The listing builds one solid part. Answer for the finished solid, in the listing's coordinates (mm). A direction names the side the tool comes from. Round coordinates to 2 decimals unless told otherwise and drop trailing zeros. Order: outer loops, then holes, each group sorted by start corner. A loop starts at its lowest first (then second) coordinate and runs counter-clockwise, first axis right, second up. Notation, with made-up numbers: (29.25, 43) -> (41.25, 43) arc R33 cw to (41.25, 73) -> close; hole circle Ø8 at (64.25, 24.5). An arc over 180 degrees is marked (long way). Answer in a Markdown table with one row per item. Add a question column.
```python
from build123d import *

# Parameters (mm, degrees)
F1_DEPTH = 50.8
F5_DEPTH = 1.27
F6_DEPTH = 1.27
F9_DEPTH = 1.27


with BuildPart() as f1:
    # F0 (on Right) → F1 (new body)
    with BuildSketch(Plane.YZ):
        with BuildLine():
            Line((8.528198, 60.317617), (-8.218083, -23.103662))
            ThreePointArc((-8.218083, -23.103662), (-25.79917, -21.313188), (-40.780291, -11.939476))
            Line((-40.780291, -11.939476), (-40.780291, -36.438663))
            Line((-40.780291, -36.438663), (49.153432, -36.438663))
            Line((49.153432, -36.438663), (49.153432, 60.317617))
            Line((49.153432, 60.317617), (8.528198, 60.317617))
        make_face()
    extrude(amount=F1_DEPTH)

    # F4 (on face) → F5 (join)
    with BuildSketch(Plane.XZ.offset(40.780291)):
        with BuildLine():
            ThreePointArc((33.516739, -31.78544), (45.164839, -24.573186), (33.516739, -17.360933))
            Line((33.516739, -17.360933), (33.516739, -31.78544))
        make_face()
        with BuildLine():
            Line((37.21533, -28.086847), (37.21533, -21.984173))
            ThreePointArc((37.21533, -21.984173), (40.963246, -25.03551), (37.21533, -28.086847))
        make_face(mode=Mode.SUBTRACT)
    extrude(amount=F5_DEPTH)

    # F3 (on face) → F6 (join)
    with BuildSketch(Plane.XZ.offset(40.780291)):
        Polygon((21.440968, -17.885948), (17.044695, -32.393657), (21.440968, -32.393657), (21.440968, -29.343316), (25.225146, -29.343316), (26.361415, -33.509634), (30.453332, -32.393657), (26.496684, -17.885948), align=None)
    extrude(amount=F6_DEPTH)

    # F8 (on face) → F9 (join)
    with BuildSketch(Plane.XZ.offset(40.780291)):
        with BuildLine():
            ThreePointArc((3.46116, -32.851707), (13.814214, -25.248081), (3.46116, -17.644456))
            Line((3.46116, -17.644456), (3.46116, -32.851707))
        make_face()
        with BuildLine():
            Line((6.277318, -22.336844), (6.277318, -22.15031))
            ThreePointArc((6.277318, -22.15031), (10.155551, -25.341956), (6.277318, -28.533602))
            Line((6.277318, -28.533602), (6.277318, -27.643853))
            ThreePointArc((6.277318, -27.643853), (6.166951, -27.608621), (6.058155, -27.5688))
            Line((6.058155, -27.5688), (6.058155, -22.411896))
            ThreePointArc((6.058155, -22.411896), (6.166951, -22.372076), (6.277318, -22.336844))
        make_face(mode=Mode.SUBTRACT)
    extrude(amount=F9_DEPTH)


solid = f1.part
```
1. Each of these flat-tipped pins is pushed along its axis until it touches: pin 1 (5 mm diameter, centred on x = 39, z = 39.5, fed in from -Y); pin 2 (1.4 mm diameter, centred on x = 23, y = -41, fed in from +Z); pin 3 (2 mm diameter, centred on x = 9, z = -25.5, fed in from -Y). Where does it stop, or does it pass through?
2. The mould has two halves that part along X. Classify faces 4 (the flat face through (25, 4, -36.439)), 5 (the flat face through (0, 24, 2)), 6 (the flat face through (39, -40.78, -25)): released by +X, released by -X, zero draft, split by the parting line, or undercut.
3. The part is cut by section D-D (z = 43). Give the vertices of the cut face in (x, y), then the cut area to 3 significant figures.
4. The part is cut by section B-B (x = 23.5). Give the vertices of the cut face in (y, z).
5. For faces 1 (the cylindrical face through (40.962, -41.406, -24.958)), 2 (the flat face through (19.274, -41.406, -25.038)), 3 (the flat face through (50.8, 24, 2)), determine the directions among +Z, -Z, +X, -X, +Y, -Y from which every point of the face is accessible in a straight line to the end or side of a thin tool.
6. The part is cut by section C-C (x = 8). Give the vertices of the cut face in (y, z).
7. Straight lines are drawn through the part: line 1 along Y through (x, z) = (16, -32); line 2 along Z through (x, y) = (37.5, -14.5); line 3 along Y through (x, z) = (28, -20). For each, find the intervals that lie inside material, in ascending order.
8. The part is cut by section A-A (z = -20). Give the vertices of the cut face in (x, y), then the cut area to 3 significant figures.
Report:
| question | item | result |
|---|---|---|
| 1 | pin 1 | stops at y = 3.85 |
| 1 | pin 2 | stops at z = -11.94 |
| 1 | pin 3 | stops at y = -40.78 |
| 2 | face 4 | zero draft |
| 2 | face 5 | released by -X |
| 2 | face 6 | undercut |
| 3 | outline | (0, 5.05) -> (50.8, 5.05) -> (50.8, 49.15) -> (0, 49.15) -> close |
| 3 | area | 2,240 mm^2 |
| 4 | outline | (-42.05, -29.34) -> (-40.78, -29.34) -> (-40.78, -36.44) -> (49.15, -36.44) -> (49.15, 60.32) -> (8.53, 60.32) -> (-8.22, -23.1) arc R38.96 cw to (-40.78, -11.94) -> (-40.78, -17.89) -> (-42.05, -17.89) -> close |
| 5 | face 1 | -Y |
| 5 | face 2 | +Z, -Y |
| 5 | face 3 | +Z, -Z, +X, +Y, -Y |
| 6 | outline | (-42.05, -32.92) -> (-40.78, -32.92) -> (-40.78, -36.44) -> (49.15, -36.44) -> (49.15, 60.32) -> (8.53, 60.32) -> (-8.22, -23.1) arc R38.96 cw to (-40.78, -11.94) -> (-40.78, -17.58) -> (-42.05, -17.58) -> (-42.05, -22.28) -> (-40.78, -22.28) -> (-40.78, -28.4) -> (-42.05, -28.4) -> close |
| 7 | line 1 | y = -40.78 to 49.15 |
| 7 | line 2 | z = -36.44 to -23.4 |
| 7 | line 3 | y = -40.78 to -29.12, -7.6 to 49.15 |
| 8 | outline | (0, -40.78) -> (3.46, -40.78) -> (3.46, -42.05) -> (11.84, -42.05) -> (11.84, -40.78) -> (20.8, -40.78) -> (20.8, -42.05) -> (27.07, -42.05) -> (27.07, -40.78) -> (33.52, -40.78) -> (33.52, -42.05) -> (43.74, -42.05) -> (43.74, -40.78) -> (50.8, -40.78) -> (50.8, -29.12) -> (0, -29.12) -> close; (0, -7.6) -> (50.8, -7.6) -> (50.8, 49.15) -> (0, 49.15) -> close |
| 8 | area | 3,510 mm^2 |
